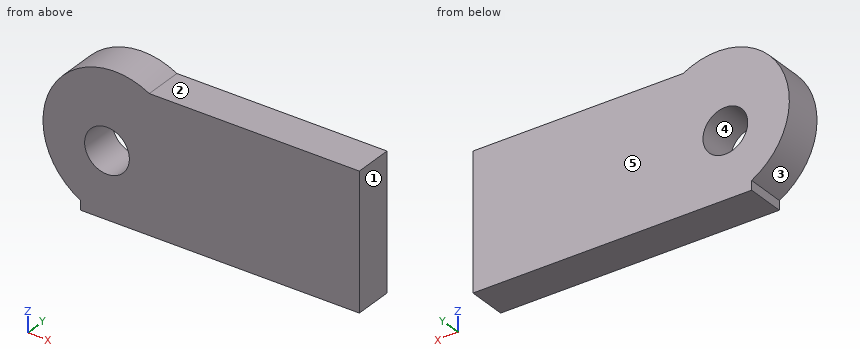
```python
from build123d import *

# Parameters (mm, degrees)
F0_R     = 14.661105288
F1_DEPTH = 25.4


with BuildPart() as f1:
    # F0 (on Front) → F1 (new body)
    with BuildSketch(Plane.XZ):
        with BuildLine():
            Line((-122.9979321361, -31.1395347035), (-122.9979321361, 51.2862093747))
            Line((-122.9979321361, 51.2862093747), (-78.072603986, 51.2862093747))
            ThreePointArc((-78.072603986, 51.2862093747), (-141.9933466372, 32.6696487834), (-122.9979321361, -31.1395347035))
        make_face()
        with BuildLine():
            Line((-78.072603986, 51.2862093747), (-122.9979321361, 51.2862093747))
            Line((-122.9979321361, 51.2862093747), (-122.9979321361, -31.1395347035))
            ThreePointArc((-122.9979321361, -31.1395347035), (-76.693666618, -30.0800117713), (-53.8420287336, 10.2065894753))
            ThreePointArc((-53.8420287336, 10.2065894753), (-60.3509770341, 34.0532661208), (-78.072603986, 51.2862093747))
        make_face()
        with Locations((-105.7746484876, 5.8953254484)):
            Circle(F0_R, mode=Mode.SUBTRACT)
        with BuildLine():
            Line((59.5510303974, 51.2862093747), (-78.072603986, 51.2862093747))
            ThreePointArc((-78.072603986, 51.2862093747), (-60.3509770341, 34.0532661208), (-53.8420287336, 10.2065894753))
            ThreePointArc((-53.8420287336, 10.2065894753), (-76.693666618, -30.0800117713), (-122.9979321361, -31.1395347035))
            Line((-122.9979321361, -31.1395347035), (-122.9979321361, -37.2208170593))
            Line((-122.9979321361, -37.2208170593), (59.5510303974, -37.2208170593))
            Line((59.5510303974, -37.2208170593), (59.5510303974, 51.2862093747))
        make_face()
    extrude(amount=F1_DEPTH)


solid = f1.part
```
CAD build for the part. Positions are in the model's coordinates, mm. Face numbers are marked on the shaded views. A direction names the side the tool comes from. Round coordinates to 2 decimals unless told otherwise and drop trailing zeros. Order: outer loops, then holes, each group sorted by start corner. A loop starts at its lowest first (then second) coordinate and runs counter-clockwise, first axis right, second up.
Item 1: Probe line 1 along Z through (x, y) = (-15.5, -13.25); line 2 along Z through (x, y) = (-97, -14); line 3 along X through (y, z) = (-18, 17). List the from-to ranges inside material, lowest first.
Item 2: Saw through at D-D on x = -40.5. Write the cut outline in (y, z).
Item 3: Saw through at C-C on y = -6. Write the cut outline in (x, z), then the cut area to 3 significant figures.
Item 4: Tool access for the marked faces 1 and 2: list every direction of +Z, -Z, +X, -X, +Y, -Y with a clear straight run to the whole face (end or side of a thin tool).
Item 5: Pin check, flat tips, straight feed: pin 1 (1.5 mm diameter, centred on y = -8.5, z = 27, fed in from -X); pin 2 (3 mm diameter, centred on y = -10, z = -35, fed in from -X); pin 3 (12 mm diameter, centred on y = -13.5, z = 3.5, fed in from -X). Stop position of each tip, or through.
Item 6: Saw through at A-A on z = 17. Write the cut outline in (x, y), then the cut area to 3 significant figures.
Item 7: Saw through at B-B on x = -113. Write the cut outline in (y, z), then the cut area to 3 significant figures.
Item 8: Mould opens along Z. For the marked faces 3, 4 and 5 say: pulls with the +Z half, pulls with the -Z half, needs draft (parallel to the pull), parting line crosses it, or undercut.
Reported:
1. line 1: z = -37.22 to 51.29
1. line 2: z = -37.22 to -5.85, 17.64 to 56.99
1. line 3: x = -147.22 to -115.35, -96.2 to 59.55
2. outline: (-25.4, -37.22) - (0, -37.22) - (0, 51.29) - (-25.4, 51.29) - close
3. outline: (-123, -37.22) - (59.55, -37.22) - (59.55, 51.29) - (-78.07, 51.29) arc R46.94 ccw (long way) to (-123, -31.14) - close; hole circle Ø29.32 at (-105.77, 5.9)
3. area: 17,100 mm2
4. face 1: +Z, -Z, +X, +Y, -Y
4. face 2: +Z, +X, +Y, -Y
5. pin 1: stops at x = -144.89
5. pin 2: stops at x = -123
5. pin 3: stops at x = -147.71
6. outline: (-147.22, -25.4) - (-115.35, -25.4) - (-115.35, 0) - (-147.22, 0) - close; (-96.2, -25.4) - (59.55, -25.4) - (59.55, 0) - (-96.2, 0) - close
6. area: 4,770 mm2
7. outline: (-25.4, -37.22) - (0, -37.22) - (0, -6.86) - (-25.4, -6.86) - close; (-25.4, 18.65) - (0, 18.65) - (0, 55.53) - (-25.4, 55.53) - close
7. area: 1,710 mm2
8. face 3: parting line crosses it
8. face 4: undercut
8. face 5: needs draft
